```python
from build123d import *
from build123d.topology import SkipClean

# Parameters (mm, degrees)
ESBO_O1_R                     = 40
RESSALTO_EXTRUS_O1_DEPTH      = 4
ESBO_O2_R                     = 2.1
CORTE_EXTRUS_O1_DEPTH         = 4
ESBO_O3_R                     = 12.5
ESBO_O3_R_2                   = 2.1
RESSALTO_EXTRUS_O2_DEPTH      = 2
RESSALTO_EXTRUS_O3_DEPTH      = 3
RESSALTO_EXTRUS_O3_DEPTH_BACK = 9
ESBO_O4_R                     = 2.75


with BuildPart() as part:
    # Esbo_o1 → Ressalto-extrus_o1 (new body)
    with BuildSketch(Plane(origin=(0, 0, 0), x_dir=(1, 0, 0), z_dir=(0, 1, 0))):
        with Locations(Location((0, 0, 0), (0, 0, 270))):
            Circle(ESBO_O1_R)
        with BuildLine():
            Line((-9.356601718, -8.288787866), (-24.640393972, -17.112889438))
            ThreePointArc((-24.640393972, -17.112889438), (0, -30), (24.640393972, -17.112889438))
            Line((24.640393972, -17.112889438), (9.356601718, -8.288787866))
            ThreePointArc((9.356601718, -8.288787866), (0, -12.5), (-9.356601718, -8.288787866))
        make_face(mode=Mode.SUBTRACT)
        with BuildLine():
            Line((-11.856601718, -3.958660847), (-27.140393972, -12.782762419))
            ThreePointArc((-27.140393972, -12.782762419), (-25.980762114, 15), (-2.5, 29.895651858))
            Line((-2.5, 29.895651858), (-2.5, 12.247448714))
            ThreePointArc((-2.5, 12.247448714), (-10.825317547, 6.25), (-11.856601718, -3.958660847))
        make_face(mode=Mode.SUBTRACT)
        with BuildLine():
            Line((2.5, 12.247448714), (2.5, 29.895651858))
            ThreePointArc((2.5, 29.895651858), (25.980762114, 15), (27.140393972, -12.782762419))
            Line((27.140393972, -12.782762419), (11.856601718, -3.958660847))
            ThreePointArc((11.856601718, -3.958660847), (10.825317547, 6.25), (2.5, 12.247448714))
        make_face(mode=Mode.SUBTRACT)
    extrude(amount=RESSALTO_EXTRUS_O1_DEPTH)

    # Esbo_o2 → Corte-extrus_o1 (cut)
    with BuildSketch(Plane(origin=(0, 4, 0), x_dir=(1, 0, 0), z_dir=(0, 1, 0))):
        with Locations(Location((0, 0, 0), (0, 0, 270))):
            Circle(ESBO_O2_R)
    extrude(amount=-CORTE_EXTRUS_O1_DEPTH, mode=Mode.SUBTRACT)

    # Esbo_o3 → Ressalto-extrus_o2 (add)
    with SkipClean():  # the faces are left unmerged after this step: merging them gives an invalid solid
        with BuildSketch(Plane(origin=(0, 4, 0), x_dir=(1, 0, 0), z_dir=(0, 1, 0))):
            with Locations(Location((0, 0, 0), (0, 0, 78.463040967))):
                Circle(ESBO_O3_R)
            with Locations(Location((0, 0, 0), (0, 0, 270))):
                Circle(ESBO_O3_R_2, mode=Mode.SUBTRACT)
        extrude(amount=RESSALTO_EXTRUS_O2_DEPTH)

    # Esbo_o4 → Ressalto-extrus_o3 (add, two sides: drawn at the far end of the back side and taken through both)
    with SkipClean():  # the faces are left unmerged after this step: merging them gives an invalid solid
        with BuildSketch(Plane(origin=(0, 6, 0), x_dir=(1, 0, 0), z_dir=(0, 1, 0)).offset(-RESSALTO_EXTRUS_O3_DEPTH_BACK)):
            with Locations(Location((0, 8, 0), (0, 0, 270))):
                Circle(ESBO_O4_R)
            with Locations(Location((8, 0, 0), (0, 0, 270))):
                Circle(ESBO_O4_R)
            with Locations(Location((0, -8, 0), (0, 0, 270))):
                Circle(ESBO_O4_R)
            with Locations(Location((-8, 0, 0), (0, 0, 270))):
                Circle(ESBO_O4_R)
        extrude(amount=RESSALTO_EXTRUS_O3_DEPTH + RESSALTO_EXTRUS_O3_DEPTH_BACK)


solid = part.part
```
For this review, take the finished solid that the model builds, in its own axes (mm). A direction names the side the tool comes from. Coordinates: 2 decimals unless noted, no trailing zeros. Write each loop counter-clockwise with the first axis right and the second up, starting at its lowest first coordinate (ties: lowest second). Pieces come first, ordered by that corner, then holes. Notation, with made-up numbers: (84.5, -6) -> (128.5, -6) arc R7 cw to (128.5, 2) -> close; hole circle Ø7 at (87.25, 81.5). An arc over 180 degrees is marked (long way). Put each result on its own line as item: value.
Q1. Take a section at C-C, the plane x = -8. State the section outline as (y, z) points, then the cut area to 3 significant figures.
From the geometry:
outline: (-3, -2.75) -> (0, -2.75) -> (0, -9.6) -> (6, -9.6) -> (6, -2.75) -> (9, -2.75) -> (9, 2.75) -> (6, 2.75) -> (6, 9.6) -> (0, 9.6) -> (0, 2.75) -> (-3, 2.75) -> close; (0, -39.19) -> (4, -39.19) -> (4, -28.91) -> (0, -28.91) -> close; (0, 28.91) -> (4, 28.91) -> (4, 39.19) -> (0, 39.19) -> close
area: 230 mm2
Q2. Take a section at B-B, the plane z = -8. State the section outline as (x, y) points, then the cut area to 3 significant figures.
From the geometry:
outline: (-39.19, 0) -> (-28.91, 0) -> (-28.91, 4) -> (-39.19, 4) -> close; (-9.6, 0) -> (-2.75, 0) -> (-2.75, -3) -> (2.75, -3) -> (2.75, 0) -> (9.6, 0) -> (9.6, 6) -> (2.75, 6) -> (2.75, 9) -> (-2.75, 9) -> (-2.75, 6) -> (-9.6, 6) -> close; (28.91, 0) -> (39.19, 0) -> (39.19, 4) -> (28.91, 4) -> close
area: 230 mm2
Q3. Tool access review of faces 1 (the cylindrical face through (-26.18, 1.97, -14.65)), 2 (the cylindrical face through (0.83, -1.52, 10.62)), 3 (the cylindrical face through (-1.05, 7.48, -5.46)), 4 (the flat face through (0, 9, -8)), 5 (the flat face through (-8, -3, 0)): name each direction out of +Z, -Z, +X, -X, +Y, -Y from which nothing blocks a thin tool from reaching the whole face with its end or side.
From the geometry:
face 1: +Y, -Y
face 2: -Y
face 3: +Y
face 4: +Z, -Z, +X, -X, +Y
face 5: +Z, -Z, +X, -X, -Y
Q4. Take a section at D-D, the plane y = -1.75. State the section outline as (x, z) points.
From the geometry:
outline: circle Ø5.5 at (-8, 0); circle Ø5.5 at (0, -8); circle Ø5.5 at (0, 8); circle Ø5.5 at (8, 0)
Q5. Take a section at A-A, the plane z = 0. Count the separate pieces of the cut face and the enclosed holes in it, then the cut area to 3 significant figures.
From the geometry:
separate pieces: 4
enclosed holes: 0
area: 271 mm2
Q6. Clearance check with flat-ended pins moving along their axes: pin 1 Ø5 at (x, z) = (0, 0) entering from +Y; pin 2 Ø3 at (x, y) = (27.5, -1) entering from +Z; pin 3 Ø6 at (x, y) = (-20, -1.5) entering from -Z; pin 4 Ø1.5 at (x, z) = (8.5, 27) entering from +Y. State where each tip first meets the part, or that it passes through.
From the geometry:
pin 1: stops at y = 6
pin 2: stops at z = 30.07
pin 3: stops at z = -36.02
pin 4: passes through
Q7. Wall thickness on L1, parallel to X at y = 2, z = 0; L2, parallel to X at y = 4.7, z = 0; L3, parallel to Z at x = -22, y = 2.5: over which ranges is each line inside the solid? List them lowest first.
From the geometry:
L1: x = -40 to -30, -12.5 to -2.1, 2.1 to 12.5, 30 to 40
L2: x = -12.5 to -2.1, 2.1 to 12.5
L3: z = -33.41 to -20.4, 9.81 to 15.59, 20.4 to 33.41
Q8. The part is to be moulded in two halves that separate along Z. For faces 6 (the cylindrical face through (-10.685, -1.521, -0.596)), 7 (the cylindrical face through (-1.05, -1.52, -5.46)), 8 (the flat face through (0, -3, 8)), say which applies: +Z half, -Z half, draft (parallel to the pull), parting line (faces both ways), or undercut.
From the geometry:
face 6: parting line
face 7: undercut
face 8: draft
